from build123d import *

# Parameters (mm, degrees)
F0_W     = 1000
F0_H     = 750
F1_DEPTH = 40
F2_W     = 40
F2_H     = 40
F3_DEPTH = 780
F4_W     = 40
F4_H     = 40
F5_DEPTH = 670
F6_W     = 40
F6_H     = 40
F7_DEPTH = 670
F8_W     = 40
F8_H     = 40
F9_DEPTH = 920


with BuildPart() as f1:
    # F0 (on Top) → F1 (new body)
    with BuildSketch(Plane.XY):
        Rectangle(F0_W, F0_H)
        Polygon((0, 335), (460, 335), (460, -335), (0, -335), (-460, -335), (-460, 335), align=None, mode=Mode.SUBTRACT)
    extrude(amount=F1_DEPTH)

    # F2 (on face) → F3 (join)
    with BuildSketch(Plane(origin=(0, 0, 0), x_dir=(1, 0, 0), z_dir=(0, 0, -1))):
        with Locations((-480, -355)):
            Rectangle(F2_W, F2_H)
        with Locations((-480, 355)):
            Rectangle(F2_W, F2_H)
        with Locations((480, 355)):
            Rectangle(F2_W, F2_H)
        with Locations((480, -355)):
            Rectangle(F2_W, F2_H)
    extrude(amount=F3_DEPTH)

    # F4 (on face) → F5 (join)
    with BuildSketch(Plane.XZ.offset(-335)):
        with Locations((-480, -560)):
            Rectangle(F4_W, F4_H)
    extrude(amount=F5_DEPTH)

    # F6 (on face) → F7 (join)
    with BuildSketch(Plane.XZ.offset(-335)):
        with Locations((480, -560)):
            Rectangle(F6_W, F6_H)
    extrude(amount=F7_DEPTH)

    # F8 (on face) → F9 (join)
    with BuildSketch(Plane(origin=(460, 0, 0), x_dir=(0, -1, 0), z_dir=(-1, 0, 0))):
        with Locations((0, -560)):
            Rectangle(F8_W, F8_H)
    extrude(amount=F9_DEPTH)


solid = f1.part
Could you check a few things on this model? Use its own coordinates, in mm. A direction names the side the tool comes from. Round coordinates to 2 decimals unless told otherwise and drop trailing zeros. Write each loop counter-clockwise with the first axis right and the second up, starting at its lowest first coordinate (ties: lowest second). Pieces come first, ordered by that corner, then holes. Notation, with made-up numbers: (-39, 53.25) -> (-5, 53.25) arc R29 ccw to (-5, 76.25) -> close; hole circle Ø11 at (81, 52). An arc over 180 degrees is marked (long way). Use a Markdown table: item, result.
1. If we section it at A-A (x = 377.5): List the corners of the cut face in (y, z) for me, then the cut area to 3 significant figures.
Answer key:
| item | result |
|---|---|
| outline | (-375, 0) -> (-335, 0) -> (-335, 40) -> (-375, 40) -> close; (-20, -580) -> (20, -580) -> (20, -540) -> (-20, -540) -> close; (335, 0) -> (375, 0) -> (375, 40) -> (335, 40) -> close |
| area | 4,800 mm^2 |
2. For pin 1 Ø12 at (x, y) = (73.5, 346.5) entering from -Z; pin 2 Ø12 at (x, z) = (-106.5, -562) entering from -Y; pin 3 Ø12 at (x, y) = (-480, 96) entering from -Z, each with a flat end and sliding along its axis, tell me the tip position at first contact or that it passes through.
Answer key:
| item | result |
|---|---|
| pin 1 | stops at z = 0 |
| pin 2 | stops at y = -20 |
| pin 3 | stops at z = -580 |
3. If we section it at B-B (z = -75.5): List the corners of the cut face in (x, y) for me.
Answer key:
| item | result |
|---|---|
| outline | (-500, -375) -> (-460, -375) -> (-460, -335) -> (-500, -335) -> close; (-500, 335) -> (-460, 335) -> (-460, 375) -> (-500, 375) -> close; (460, -375) -> (500, -375) -> (500, -335) -> (460, -335) -> close; (460, 335) -> (500, 335) -> (500, 375) -> (460, 375) -> close |
4. If we section it at C-C (y = 265.5): List the corners of the cut face in (x, z) for me, then the cut area to 3 significant figures.
Answer key:
| item | result |
|---|---|
| outline | (-500, -580) -> (-460, -580) -> (-460, -540) -> (-500, -540) -> close; (-500, 0) -> (-460, 0) -> (-460, 40) -> (-500, 40) -> close; (460, -580) -> (500, -580) -> (500, -540) -> (460, -540) -> close; (460, 0) -> (500, 0) -> (500, 40) -> (460, 40) -> close |
| area | 6,400 mm^2 |
5. Which directions (+Z, -Z, +X, -X, +Y, -Y) give clear straight access to the entire face, cutting with the end or side of a thin tool? Please do faces 1 (the face through (6, 20, -560)), 2 (the face through (460, -341, -446)), 3 (the face through (460, 343, -417)).
Answer key:
| item | result |
|---|---|
| face 1 | +Z, -Z, +Y |
| face 2 | -Z, -Y |
| face 3 | -Z, +Y |
6. Please list where these lines run through material, in increasing order: probe 1 along X at (y, z) = (156, 1); probe 2 along Y at (x, z) = (89.5, -553).
Answer key:
| item | result |
|---|---|
| probe 1 | x = -500 to -460, 460 to 500 |
| probe 2 | y = -20 to 20 |
7. We'd pull the mould along X, two halves only. Please class faces 4 (the face through (480, 335, -266)), 5 (the face through (500, -57, -554)), 6 (the face through (460, 5, 20)), 7 (the face through (-500, 85, -550)): +X half, -X half, draft (parallel to the pull), parting line (faces both ways), or undercut.
Answer key:
| item | result |
|---|---|
| face 4 | draft |
| face 5 | +X half |
| face 6 | undercut |
| face 7 | -X half |
